Model file for the job. Use its own axes, mm. A direction names the side the tool comes from. Round coordinates to 2 decimals unless told otherwise and drop trailing zeros. Loops run counter-clockwise (first coordinate to the right, second up) from the corner with the lowest first, then second, coordinate; pieces in that order, holes last.
from build123d import *

# Parameters (mm, degrees)
F0_W     = 112
F0_H     = 125
F1_DEPTH = 8
F2_DEPTH = 10
F0_W_2   = 176
F3_DEPTH = 12


with BuildPart() as f1:
    # F0 (on Front) → F1 (new body)
    with BuildSketch(Plane.XZ):
        with Locations((-144, 250)):
            Rectangle(F0_W, F0_H)
        with Locations((144, 250)):
            Rectangle(F0_W, F0_H)
    extrude(amount=F1_DEPTH)

    # F0 (on Front) → F2 (join)
    with BuildSketch(Plane.XZ):
        Polygon((-200, 187.5), (-200, -312.5), (200, -312.5), (200, 187.5), (88, 187.5), (-88, 187.5), align=None)
    extrude(amount=F2_DEPTH)

    # F0 (on Front) → F3 (join)
    with BuildSketch(Plane.XZ):
        with Locations((0, 250)):
            Rectangle(F0_W_2, F0_H)
    extrude(amount=F3_DEPTH)


solid = f1.part
Q1. Slice it at A-A on z = 261. Give the cut face in (x, y), plus the area to 3 significant figures.
Q2. Flat gauge pins, fed straight in: P1, Ø3, axis at x = 34.5, z = -180, coming from the -Y side; P2, Ø1.2, axis at y = -10, z = 274, coming from the +X side; P3, Ø0.6, axis at x = 119, y = -9, coming from the +Z side. Where does each tip first touch, or does it go through?
Q3. Probe line 1 (Y direction, x = 160, z = 18); line 2 (Z direction, x = 101, y = -9.5); line 3 (Y direction, x = 163.5, z = 250). List the from-to ranges inside material, lowest first.
Q4. Tool access for faces 1 (the face through (143, -8, 251)), 2 (the face through (-145, -8, 251)), 3 (the face through (-3, -10, -59)), 4 (the face through (-3, -5, 312.5)): list every direction of +Z, -Z, +X, -X, +Y, -Y with a clear straight run to the whole face (end or side of a thin tool).
Q5. Slice it at C-C on x = -26. Give the cut face in (y, z).
Q6. Slice it at D-D on z = 25.5. Give the cut face in (x, y).
Q7. Slice it at B-B on x = -161. Give the cut face in (y, z).
Reply:
1. outline: (-200, -8) - (-88, -8) - (-88, -12) - (88, -12) - (88, -8) - (200, -8) - (200, 0) - (-200, 0) - close
1. area: 3,900 mm2
2. P1: stops at y = -10
2. P2: stops at x = 88
2. P3: stops at z = 187.5
3. line 1: y = -10 to 0
3. line 2: z = -312.5 to 187.5
3. line 3: y = -8 to 0
4. face 1: +Z, +X, -Y
4. face 2: +Z, -X, -Y
4. face 3: -Z, +X, -X, -Y
4. face 4: +Z, +X, -X, +Y, -Y
5. outline: (-12, 187.5) - (-10, 187.5) - (-10, -312.5) - (0, -312.5) - (0, 312.5) - (-12, 312.5) - close
6. outline: (-200, -10) - (200, -10) - (200, 0) - (-200, 0) - close
7. outline: (-10, -312.5) - (0, -312.5) - (0, 312.5) - (-8, 312.5) - (-8, 187.5) - (-10, 187.5) - close
